from build123d import *

# Parameters (mm, degrees)
SKETCH1_W           = 20
SKETCH1_H           = 155
BOSS_EXTRUDE1_DEPTH = 4
SKETCH2_W           = 20
SKETCH2_H           = 4
BOSS_EXTRUDE3_DEPTH = 50
RIB2_REACH          = 96.986
SKETCH7_WALL_W      = 290.205463948
SKETCH7_WALL_H      = 4
SKETCH8_W           = 20
SKETCH8_H           = 3
BOSS_EXTRUDE4_DEPTH = 3.5
BOSS_EXTRUDE6_DEPTH = 3
SKETCH10_W          = 10
SKETCH10_H          = 3
BOSS_EXTRUDE7_DEPTH = 7.5
SKETCH12_R          = 1.75
CUT_EXTRUDE1_DEPTH  = 10


with BuildPart() as part:
    # Sketch1 → Boss-Extrude1 (new body)
    with BuildSketch(Plane.XY):
        Rectangle(SKETCH1_W, SKETCH1_H)
    extrude(amount=BOSS_EXTRUDE1_DEPTH)

    # Sketch2 → Boss-Extrude3 (add)
    with BuildSketch(Plane.XY.offset(4)):
        with Locations((0, -75.5)):
            Rectangle(SKETCH2_W, SKETCH2_H)
    extrude(amount=BOSS_EXTRUDE3_DEPTH)

    # Sketch7 wall → Rib2 (add, up to next)
    with BuildSketch(Plane(origin=(0, -26, 16.5), x_dir=(0, 0.967074537263, -0.25449329928), z_dir=(0, 0.25449329928, 0.967074537263)), mode=Mode.PRIVATE) as rib2_sk1:
        Rectangle(SKETCH7_WALL_W, SKETCH7_WALL_H)
    rib2_tool1 = extrude(rib2_sk1.sketch, amount=-RIB2_REACH, mode=Mode.PRIVATE) - part.part
    add(rib2_tool1.solids().sort_by_distance((0, -26, 16.5))[0])

    # Sketch8 → Boss-Extrude4 (add)
    with BuildSketch(Plane.XY.offset(4)):
        with Locations((0, 76)):
            Rectangle(SKETCH8_W, SKETCH8_H)
    extrude(amount=BOSS_EXTRUDE4_DEPTH)

    # Sketch9 → Boss-Extrude6 (add)
    with BuildSketch(Plane.XY.offset(7.5)):
        Polygon((-21.75, 74.5), (0, 74.5), (21.75, 74.5), (21.75, 79.5), (-21.75, 79.5), align=None)
    extrude(amount=BOSS_EXTRUDE6_DEPTH)

    # Sketch10 → Boss-Extrude7 (add)
    with BuildSketch(Plane(origin=(0, 0, 7.5), x_dir=(-1, 0, 0), z_dir=(0, 0, -1))):
        with Locations((16.75, 76)):
            Rectangle(SKETCH10_W, SKETCH10_H)
        with Locations((-16.75, 76)):
            Rectangle(SKETCH10_W, SKETCH10_H)
    extrude(amount=BOSS_EXTRUDE7_DEPTH)

    # Sketch12 → Cut-Extrude1 (cut)
    with BuildSketch(Plane(origin=(0, 77.5, 0), x_dir=(1, 0, 0), z_dir=(0, 1, 0))):
        with Locations(Location((-17.75, -3.5, 0), (0, 0, 270))):
            Circle(SKETCH12_R)
        with Locations(Location((17.75, -3.5, 0), (0, 0, 270))):
            Circle(SKETCH12_R)
    extrude(amount=-CUT_EXTRUDE1_DEPTH, mode=Mode.SUBTRACT)


solid = part.part
Read the model definition and answer for the solid it produces. Units are mm, in the model's axes. A direction names the side the tool comes from. Give positions to 0.01 mm unless a question says otherwise; leave off trailing zeros. Write each loop counter-clockwise with the first axis right and the second up, starting at its lowest first coordinate (ties: lowest second). Pieces come first, ordered by that corner, then holes. Notation, with made-up numbers: (21, 64.25) - (28, 64.25) arc R33 cw to (28, 95.25) - close; hole circle Ø9 at (-32, 0.25). An arc over 180 degrees is marked (long way). Use CSV: the item, a comma, the result in double quotes. Start each with the question number.
Item 1: The part is cut by section B-B, the plane z = 18.5. Give the vertices of the cut face in (x, y), and give its area (3 significant figures).
Item 2: For faces 1 (the flat face through (-11.75, 76, 4)), 2 (the flat face through (0, 77.5, 4)), 3 (the flat face through (-2.4, 1.5, 4)), 4 (the flat face through (-21.75, 76, 6)), 5 (the flat face through (-17, 76, 0)), determine the directions among +Z, -Z, +X, -X, +Y, -Y from which every point of the face is accessible in a straight line to the end or side of a thin tool.
Item 3: Consider line 1 (X direction, y = 76.55, z = 3.5); line 2 (X direction, y = 75, z = 3); line 3 (Y direction, x = 4.5, z = 10). Determine where each line is inside the solid, lowest interval first.
Item 4: The part is cut by section A-A, the plane x = -17.75. Give the vertices of the cut face in (y, z), and give its area (3 significant figures).
Item 5: The part is cut by section D-D, the plane z = 25. Give the vertices of the cut face in (x, y).
Item 6: The mould has two halves that part along Y. Classify faces 6 (the flat face through (-15.6, 77.5, 3.8)), 7 (the flat face through (-2, -39, 13)), 8 (the flat face through (-0.028, -26.665, 16.675)), 9 (the flat face through (17, 76, 0)): pulls with the +Y half, pulls with the -Y half, needs draft (parallel to the pull), parting line crosses it, or undercut.
Item 7: Flat-ended cylindrical pins translate along their axes: P1, Ø5.5, axis at x = 1, y = 76, coming from the +Z side; P2, Ø4, axis at x = 17.75, z = 3.5, coming from the -Y side; P3, Ø10, axis at x = -3, y = 17, coming from the +Z side. Find the tip coordinate at first contact, or state that the pin passes through.
Item 8: The part is cut by section C-C, the plane y = 37. Give the vertices of the cut face in (x, z).
Taken from the geometry:
1,outline,"(-10, -77.5) - (10, -77.5) - (10, -73.5) - (2, -73.5) - (2, -33.6) - (-2, -33.6) - (-2, -73.5) - (-10, -73.5) - close"
1,area,"240 mm2"
2,face 1,"-Z, +Y, -Y"
2,face 2,"-Z, +X, -X, +Y"
2,face 3,"+Z"
2,face 4,"+Z, -Z, -X, +Y, -Y"
2,face 5,"-Z, +X, -X, +Y, -Y"
3,line 1,"-21.75 to -19.5, -16 to -11.75, -10 to 10, 11.75 to 16, 19.5 to 21.75"
3,line 2,"-21.75 to -19.43, -16.07 to -11.75, -10 to 10, 11.75 to 16.07, 19.43 to 21.75"
3,line 3,"-77.5 to -73.5, 74.5 to 79.5"
4,outline,"(74.5, 0) - (77.5, 0) - (77.5, 1.75) - (74.5, 1.75) - close; (74.5, 5.25) - (77.5, 5.25) - (77.5, 7.5) - (79.5, 7.5) - (79.5, 10.5) - (74.5, 10.5) - close"
4,area,"27.0 mm2"
5,outline,"(-10, -77.5) - (10, -77.5) - (10, -73.5) - (2, -73.5) - (2, -58.3) - (-2, -58.3) - (-2, -73.5) - (-10, -73.5) - close"
6,face 6,"pulls with the +Y half"
6,face 7,"undercut"
6,face 8,"undercut"
6,face 9,"needs draft"
7,P1,"z = 10.5"
7,P2,"y = 74.5"
7,P3,"z = 6.47"
8,outline,"(-10, 0) - (10, 0) - (10, 4) - (-10, 4) - close"
